```python
from build123d import *

# Parameters (mm, degrees)
SKETCH1_R             = 31
SKETCH1_R_2           = 26
BOSS_EXTRUDE1_DEPTH   = 7
SKETCH2_R             = 31
SKETCH2_R_2           = 25
BOSS_EXTRUDE3_DEPTH   = 10
SKETCH3_R             = 31
SKETCH3_R_2           = 26
BOSS_EXTRUDE4_DEPTH   = 7
FILLET1_R             = 0.3
SKETCH4_W             = 80
SKETCH4_H             = 80
SKETCH4_R             = 31
BOSS_EXTRUDE5_DEPTH   = 5
FILLET2_R             = 2
M6X1_0_TAPPED_HOLE1_D = 5
SKETCH7_W             = 10
SKETCH7_H             = 5
BOSS_EXTRUDE6_DEPTH   = 80
FILLET3_R             = 5
SKETCH8_W             = 20
SKETCH8_H             = 5
BOSS_EXTRUDE7_DEPTH   = 80
M6X1_0_TAPPED_HOLE2_D = 5


with BuildPart() as part:
    # Sketch1 → Boss-Extrude1 (new body)
    with BuildSketch(Plane.XY):
        Circle(SKETCH1_R)
        Circle(SKETCH1_R_2, mode=Mode.SUBTRACT)
    extrude(amount=BOSS_EXTRUDE1_DEPTH)

    # Sketch2 → Boss-Extrude3 (add)
    with BuildSketch(Plane.XY.offset(7)):
        Circle(SKETCH2_R)
        Circle(SKETCH2_R_2, mode=Mode.SUBTRACT)
    extrude(amount=BOSS_EXTRUDE3_DEPTH)

    # Sketch3 → Boss-Extrude4 (add)
    with BuildSketch(Plane.XY.offset(17)):
        Circle(SKETCH3_R)
        Circle(SKETCH3_R_2, mode=Mode.SUBTRACT)
    extrude(amount=BOSS_EXTRUDE4_DEPTH)

    # Fillet1
    fillet1_edges = [part.edges().sort_by_distance(p)[0] for p in [
        (-26, 0, 7),
        (-26, 0, 17),
    ]]
    fillet(fillet1_edges, radius=FILLET1_R)

    # Sketch4 → Boss-Extrude5 (add)
    with BuildSketch(Plane.XY.offset(24)):
        Rectangle(SKETCH4_W, SKETCH4_H)
        Circle(SKETCH4_R, mode=Mode.SUBTRACT)
    extrude(amount=-BOSS_EXTRUDE5_DEPTH)

    # Fillet2
    fillet2_edges = [part.edges().sort_by_distance(p)[0] for p in [
        (-31, 0, 19),
    ]]
    fillet(fillet2_edges, radius=FILLET2_R)

    # M6x1.0 Tapped Hole1 (through all)
    with Locations(Plane.XY.offset(24)):
        with Locations((-32, 27.5), (32, 27.5), (32, -27.5), (-32, -27.5)):
            Hole(M6X1_0_TAPPED_HOLE1_D / 2)

    # Sketch7 → Boss-Extrude6 (add)
    with BuildSketch(Plane(origin=(40, 0, 0), x_dir=(0, 0, -1), z_dir=(1, 0, 0))):
        with Locations((-24, 42.5)):
            Rectangle(SKETCH7_W, SKETCH7_H)
        with Locations((-24, -42.5)):
            Rectangle(SKETCH7_W, SKETCH7_H)
    extrude(amount=-BOSS_EXTRUDE6_DEPTH)

    # Fillet3
    fillet3_edges = [part.edges().sort_by_distance(p)[0] for p in [
        (0, 45, 19),
        (0, -45, 19),
    ]]
    fillet(fillet3_edges, radius=FILLET3_R)

    # Sketch8 → Boss-Extrude7 (add)
    with BuildSketch(Plane(origin=(40, 0, 0), x_dir=(0, 0, -1), z_dir=(1, 0, 0))):
        with Locations((-39, 42.5)):
            Rectangle(SKETCH8_W, SKETCH8_H)
        with Locations((-39, -42.5)):
            Rectangle(SKETCH8_W, SKETCH8_H)
    extrude(amount=-BOSS_EXTRUDE7_DEPTH)

    # M6x1.0 Tapped Hole2 (through all)
    with Locations(Plane(origin=(0, 45, 0), x_dir=(1, 0, 0), z_dir=(0, 1, 0))):
        with Locations((-22.6, -39), (22.6, -39)):
            Hole(M6X1_0_TAPPED_HOLE2_D / 2)


solid = part.part
```
For this review, take the finished solid that the model builds, in its own axes (mm). A direction names the side the tool comes from. Round coordinates to 2 decimals unless told otherwise and drop trailing zeros. Write each loop counter-clockwise with the first axis right and the second up, starting at its lowest first coordinate (ties: lowest second). Pieces come first, ordered by that corner, then holes. Notation, with made-up numbers: (77, 77.5) -> (93, 77.5) arc R23 cw to (93, 111.5) -> close; hole circle Ø7 at (88, 71). An arc over 180 degrees is marked (long way). One line per question, with ' | ' between items. Start each with the question number.
(1) Tool access review of faces 5 (the face through (-16, -21, 0)), 6 (the face through (1, 40, 37)), 7 (the face through (-20.633, -15.821, 3.303)): name each direction out of +Z, -Z, +X, -X, +Y, -Y from which nothing blocks a thin tool from reaching the whole face with its end or side.
(2) Add section C-C, the plane z = 39. Write out the cut boundary in (x, y).
(3) Insertion check: P1, Ø1.5, axis at x = -22, z = 22.5, coming from the -Y side; P2, Ø8, axis at x = 3.5, y = -22.5, coming from the +Z side; P3, Ø6, axis at x = -1.5, z = 10, coming from the +Y side. Each pin has a flat end and moves straight along its axis. Give the tip position at first contact, or say it passes through.
(4) Mouldability with a two-part tool opening along X and no side actions: class faces 1 (the face through (-1, -43, 20)), 2 (the face through (40, 7, 23)), 3 (the face through (-4.036, 30.736, 8.381)), 4 (the face through (-22.06, -42.54, 41.44)) as released by +X, released by -X, zero draft, split by the parting line, or undercut.
(5) Add section D-D, the plane x = -22.6. Give the number of separate pieces and of enclosed holes in the cut face, plus the area to 3 significant figures.
(6) Add section B-B, the plane z = 46. Write out the cut boundary in (x, y), plus the area to 3 significant figures.
(7) For line 1 along X through (y, z) = (-42.15, 39); line 2 along Y through (x, z) = (-13, 35.5); line 3 along Y through (x, z) = (-32, 21), list the stretches that pass through material, from the lowest coordinate up. Write a range as from..to.
(8) Add section A-A, the plane y = 0. Write out the cut boundary in (x, z).
Answer list:
1) face 5: -Z, +X, -X, +Y, -Y | face 6: +Z, +X, -X | face 7: -Z
2) outline: (-40, -45) -> (-25.1, -45) -> (-25.1, -40) -> (-40, -40) -> close; (-40, 40) -> (-25.1, 40) -> (-25.1, 45) -> (-40, 45) -> close; (-20.1, -45) -> (20.1, -45) -> (20.1, -40) -> (-20.1, -40) -> close; (-20.1, 40) -> (20.1, 40) -> (20.1, 45) -> (-20.1, 45) -> close; (25.1, -45) -> (40, -45) -> (40, -40) -> (25.1, -40) -> close; (25.1, 40) -> (40, 40) -> (40, 45) -> (25.1, 45) -> close
3) P1: y = -44.94 | P2: z = 24 | P3: y = 31
4) face 1: zero draft | face 2: released by +X | face 3: split by the parting line | face 4: undercut
5) separate pieces: 4 | enclosed holes: 0 | area: 875 mm²
6) outline: (-40, -45) -> (40, -45) -> (40, -40) -> (-40, -40) -> close; (-40, 40) -> (40, 40) -> (40, 45) -> (-40, 45) -> close | area: 800 mm²
7) line 1: -40..-25.1, -20.1..20.1, 25.1..40 | line 2: -45..-40, 40..45 | line 3: -44..-30, -25..25, 30..44
8) outline: (-40, 19) -> (-33, 19) arc R2 cw to (-31, 17) -> (-31, 0) -> (-26, 0) -> (-26, 6.7) arc R0.3 cw to (-25.7, 7) -> (-25, 7) -> (-25, 17) -> (-25.7, 17) arc R0.3 cw to (-26, 17.3) -> (-26, 24) -> (-40, 24) -> close; (25, 7) -> (25.7, 7) arc R0.3 cw to (26, 6.7) -> (26, 0) -> (31, 0) -> (31, 17) arc R2 cw to (33, 19) -> (40, 19) -> (40, 24) -> (26, 24) -> (26, 17.3) arc R0.3 cw to (25.7, 17) -> (25, 17) -> close
